```python
from build123d import *
from build123d.topology import SkipClean

# Parameters (mm, degrees)
BOSS_EXTRUDE1_DEPTH                                 = 10.16
CBORE_FOR_0_BINDING_HEAD_MACHINE_SCREW1_D           = 5.08
CBORE_FOR_0_BINDING_HEAD_MACHINE_SCREW1_CBORE_D     = 7.62
CBORE_FOR_0_BINDING_HEAD_MACHINE_SCREW1_CBORE_DEPTH = 1.27
SHELL1_OUTLINE_R                                    = 6.35
SHELL1_DEPTH                                        = 7.62
SHELL1_2_OUTLINE_R                                  = 6.35
SHELL1_2_OUTLINE_R_2                                = 5.08
SHELL1_2_DEPTH                                      = 6.35
CUT_EXTRUDE1_DEPTH                                  = 1.778
CUT_EXTRUDE2_DEPTH                                  = 1.778
CUT_EXTRUDE5_REACH                                  = 157.506
CUT_EXTRUDE6_REACH                                  = 157.506
CUT_EXTRUDE3_DEPTH                                  = 156.506301159
CUT_EXTRUDE3_DEPTH_BACK                             = 156.506301159
SKETCH4_W                                           = 120.65
SKETCH4_H                                           = 5.08
SKETCH5_W                                           = 19.05
SKETCH5_H                                           = 5.08
CUT_EXTRUDE4_DEPTH                                  = 2.54
SKETCH9_W                                           = 47.752
SKETCH9_H                                           = 3.81
CUT_EXTRUDE7_DEPTH                                  = 2.413
FILLET1_R                                           = 1.27
BOSS_EXTRUDE2_DEPTH                                 = 2.54
SKETCH11_W                                          = 40.132
SKETCH11_H                                          = 1.27
CUT_EXTRUDE9_DEPTH                                  = 6.858
SKETCH20_R                                          = 6.35
SKETCH20_R_2                                        = 5.08
CUT_EXTRUDE11_DEPTH                                 = 1.27
BOSS_EXTRUDE4_START                                 = 2.159
BOSS_EXTRUDE4_DEPTH                                 = 2.159
SKETCH36_R                                          = 1.905
CUT_EXTRUDE18_DEPTH                                 = 155.437689597


# Read off the part's stored shape, not the designer's step: Shell1
with BuildPart() as part:
    # Sketch1 → Boss-Extrude1 (new body)
    with BuildSketch(Plane(origin=(0, 0, 0), x_dir=(1, 0, 0), z_dir=(0, 1, 0))):
        with BuildLine():
            Line((0, 0), (133.35, 0))
            Line((133.35, 0), (152.4, 29.21))
            Line((152.4, 29.21), (35.446425772, 29.21))
            ThreePointArc((35.446425772, 29.21), (12.577020299, 22.164640842), (-2.363095051, 3.471333333))
            ThreePointArc((-2.363095051, 3.471333333), (-2.099665053, 1.110662158), (0, 0))
        make_face()
    extrude(amount=BOSS_EXTRUDE1_DEPTH)

    # CBORE for #0 Binding Head Machine Screw1 (through all)
    with Locations(Plane(origin=(0, 10.16, 0), x_dir=(1, 0, 0), z_dir=(0, 1, 0))):
        with Locations((74.100334947, 9.652)):
            CounterBoreHole(CBORE_FOR_0_BINDING_HEAD_MACHINE_SCREW1_D / 2, CBORE_FOR_0_BINDING_HEAD_MACHINE_SCREW1_CBORE_D / 2, CBORE_FOR_0_BINDING_HEAD_MACHINE_SCREW1_CBORE_DEPTH)

    # Shell1 outline → Shell1 (cut)
    with BuildSketch(Plane(origin=(0, 0, 0), x_dir=(1, 0, 0), z_dir=(0, 1, 0))):
        with BuildLine():
            Line((150.743478261, 26.67), (35.446425772, 26.67))
            ThreePointArc((35.446425772, 26.67), (14.006358141, 20.06497579), (0, 2.54))
            Line((0, 2.54), (135.006521739, 2.54))
            Line((135.006521739, 2.54), (150.743478261, 26.67))
        make_face()
        with Locations((74.100334947, 9.652)):
            Circle(SHELL1_OUTLINE_R, mode=Mode.SUBTRACT)
    extrude(amount=SHELL1_DEPTH, mode=Mode.SUBTRACT)

    # Shell1 2 outline → Shell1 2 (cut)
    with BuildSketch(Plane(origin=(0, 0, 0), x_dir=(1, 0, 0), z_dir=(0, 1, 0))):
        with Locations((74.100334947, 9.652)):
            Circle(SHELL1_2_OUTLINE_R)
        with Locations((74.100334947, 9.652)):
            Circle(SHELL1_2_OUTLINE_R_2, mode=Mode.SUBTRACT)
    extrude(amount=SHELL1_2_DEPTH, mode=Mode.SUBTRACT)

    # Sketch2 → Cut-Extrude1 (cut)
    with BuildSketch(Plane.XY):
        Polygon((118.11, 0), (118.11, 5.08), (119.38, 5.08), (119.38, 10.16), (111.76, 10.16), (105.41, 0), align=None)
    extrude(amount=-CUT_EXTRUDE1_DEPTH, mode=Mode.SUBTRACT)

    # Sketch3 → Cut-Extrude2 (cut)
    with BuildSketch(Plane(origin=(0, 0, -29.21), x_dir=(-1, 0, 0), z_dir=(0, 0, -1))):
        Polygon((-138.43, 10.16), (-138.43, 5.08), (-137.16, 5.08), (-137.16, 0), (-124.46, 0), (-130.81, 10.16), align=None)
    extrude(amount=-CUT_EXTRUDE2_DEPTH, mode=Mode.SUBTRACT)

    # Cut-Extrude5: up to this face of the body (flat: up to its plane)
    cut_extrude5_end = Plane(part.part.faces().sort_by_distance((67.503260869, 3.81, -2.54))[0])
    # Sketch7 → Cut-Extrude5 (cut, up to the picked face)
    with BuildSketch(Plane.XY, mode=Mode.PRIVATE) as cut_extrude5_sk1:
        Polygon((135.006521739, 2.979312663), (118.11, 0), (135.006521739, 0), align=None)
    cut_extrude5_tool1 = split(extrude(cut_extrude5_sk1.sketch, amount=-CUT_EXTRUDE5_REACH, mode=Mode.PRIVATE), bisect_by=cut_extrude5_end, keep=Keep.BOTH, mode=Mode.PRIVATE)
    add(cut_extrude5_tool1.solids().sort_by(Axis((129.374348, 0.993104, 0), (0, 0, -1)))[0], mode=Mode.SUBTRACT)

    # Cut-Extrude6: up to this face of the body (flat: up to its plane)
    cut_extrude6_end = Plane(part.part.faces().sort_by_distance((93.094952017, 3.81, -26.67))[0])
    # Sketch8 → Cut-Extrude6 (cut, up to the picked face)
    with BuildSketch(Plane(origin=(0, 0, -29.21), x_dir=(-1, 0, 0), z_dir=(0, 0, -1)), mode=Mode.PRIVATE) as cut_extrude6_sk1:
        Polygon((-152.4, 2.687223186), (-137.16, 0), (-152.4, 0), align=None)
    cut_extrude6_tool1 = split(extrude(cut_extrude6_sk1.sketch, amount=-CUT_EXTRUDE6_REACH, mode=Mode.PRIVATE), bisect_by=cut_extrude6_end, keep=Keep.BOTH, mode=Mode.PRIVATE)
    add(cut_extrude6_tool1.solids().sort_by(Axis((147.32, 0.895741, -29.21), (0, 0, 1)))[0], mode=Mode.SUBTRACT)

    # Sketch4 → Cut-Extrude3 (cut, two sides: drawn at the far end of the back side and taken through both)
    with BuildSketch(Plane.XY.offset(-CUT_EXTRUDE3_DEPTH_BACK)):
        with Locations((57.785, 2.54)):
            Rectangle(SKETCH4_W, SKETCH4_H)
    extrude(amount=CUT_EXTRUDE3_DEPTH + CUT_EXTRUDE3_DEPTH_BACK, mode=Mode.SUBTRACT)

    # Sketch5 → Cut-Extrude4 (cut)
    with BuildSketch(Plane(origin=(0, 0, -29.21), x_dir=(-1, 0, 0), z_dir=(0, 0, -1))):
        with Locations((-127.635, 2.54)):
            Rectangle(SKETCH5_W, SKETCH5_H)
    extrude(amount=-CUT_EXTRUDE4_DEPTH, mode=Mode.SUBTRACT)

    # Sketch9 → Cut-Extrude7 (cut)
    with BuildSketch(Plane(origin=(0, 0, -29.21), x_dir=(-1, 0, 0), z_dir=(0, 0, -1))):
        with Locations((-99.949, 6.985)):
            Rectangle(SKETCH9_W, SKETCH9_H)
    extrude(amount=-CUT_EXTRUDE7_DEPTH, mode=Mode.SUBTRACT)

    # Fillet1
    fillet1_edges = [part.edges().sort_by_distance(p)[0] for p in [
        (145.415, 10.16, -29.21),
        (142.875, 10.16, -14.605),
        (126.365, 10.16, 0),
        (119.38, 10.16, -0.889),
        (55.88, 10.16, 0),
        (-2.099665053, 10.16, -1.110662158),
        (12.577020299, 10.16, -22.164640842),
        (83.128212886, 10.16, -29.21),
        (138.43, 10.16, -28.321),
        (133.35, 6.423611593, 0),
        (152.4, 6.423611593, -29.21),
        (0, 6.35, -2.54),
        (118.745, 5.08, 0),
        (118.11, 2.54, 0),
        (119.38, 7.62, 0),
        (137.16, 2.54, -29.21),
        (137.795, 5.08, -29.21),
        (138.43, 7.62, -29.21),
        (144.78, 1.343611593, -29.21),
        (125.73, 1.343611593, 0),
        (151.57173913, 2.541178448, -27.94),
        (134.17826087, 2.833267924, -1.27),
        (137.16, 5.08, -28.321),
        (118.11, 0, -1.27),
        (118.11, 5.08, -0.889),
        (137.16, 0, -27.94),
    ]]
    fillet(fillet1_edges, radius=FILLET1_R - 0.0001)  # a hair under: the kernel refuses the full size

    # Sketch10 → Boss-Extrude2 (add)
    with BuildSketch(Plane.XZ.offset(-7.62)):
        Polygon((79.883, -21.717), (79.883, -26.67), (112.903, -26.67), (112.903, -19.939), (110.363, -19.939), (110.363, -23.749), (105.283, -23.749), (105.283, -21.717), (102.743, -21.717), (102.743, -23.749), (100.203, -23.749), (100.203, -21.717), (97.663, -21.717), (97.663, -23.749), (95.123, -23.749), (95.123, -21.717), (92.583, -21.717), (92.583, -23.749), (90.043, -23.749), (90.043, -21.717), (87.503, -21.717), (87.503, -23.749), (84.963, -23.749), (84.963, -21.717), align=None)
    extrude(amount=BOSS_EXTRUDE2_DEPTH)

    # Sketch11 → Cut-Extrude9 (cut)
    with BuildSketch(Plane(origin=(0, 0, -26.797), x_dir=(-1, 0, 0), z_dir=(0, 0, -1))):
        with Locations((-99.949, 5.715)):
            Rectangle(SKETCH11_W, SKETCH11_H)
    extrude(amount=-CUT_EXTRUDE9_DEPTH, mode=Mode.SUBTRACT)

    # Sketch20 → Cut-Extrude11 (cut)
    with SkipClean():  # the faces are left unmerged after this step: merging them gives an invalid solid
        with BuildSketch(Plane.XZ.offset(-6.35)):
            with Locations((74.100334947, -9.652)):
                Circle(SKETCH20_R)
            with Locations(Location((74.100334947, -9.652, 0), (0, 0, 90))):
                Circle(SKETCH20_R_2, mode=Mode.SUBTRACT)
        extrude(amount=-CUT_EXTRUDE11_DEPTH, mode=Mode.SUBTRACT)

    # Sketch21 → Boss-Extrude4 (add)
    with BuildSketch(Plane.XZ.offset(-7.62).offset(BOSS_EXTRUDE4_START)):
        with BuildLine():
            Line((74.100334947, -2.54), (74.100334947, -4.572))
            ThreePointArc((74.100334947, -4.572), (73.196935106, -4.652973222), (72.322334947, -4.893311525))
            Line((72.322334947, -4.893311525), (72.322334947, -2.54))
            Line((72.322334947, -2.54), (74.100334947, -2.54))
        make_face()
        with BuildLine():
            Line((74.100334947, -14.732), (74.100334947, -26.67))
            Line((74.100334947, -26.67), (72.322334947, -26.67))
            Line((72.322334947, -26.67), (72.322334947, -14.410688475))
            ThreePointArc((72.322334947, -14.410688475), (73.196935106, -14.651026778), (74.100334947, -14.732))
        make_face()
    extrude(amount=-BOSS_EXTRUDE4_DEPTH)

    # Sketch36 → Cut-Extrude18 (cut, through all)
    with SkipClean():  # the faces are left unmerged after this step: merging them gives an invalid solid
        with BuildSketch(Plane(origin=(0, 10.16, 0), x_dir=(1, 0, 0), z_dir=(0, 1, 0))):
            with Locations(Location((0, 2.54, 0), (0, 0, 270))):
                Circle(SKETCH36_R)
        extrude(amount=-CUT_EXTRUDE18_DEPTH, mode=Mode.SUBTRACT)


solid = part.part
```
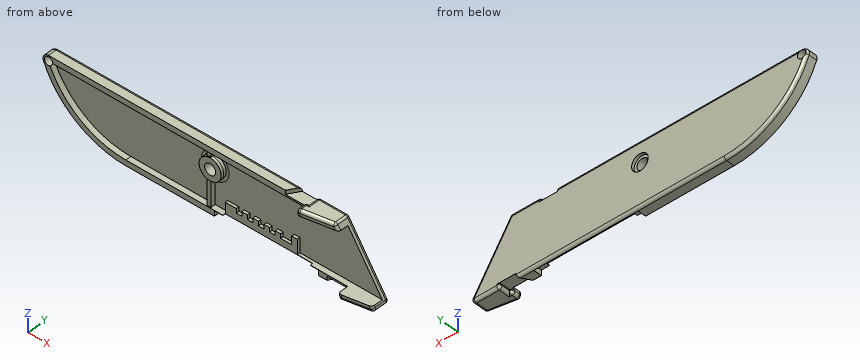
Can you work these out from the model? Positions are in its coordinate system, mm. Round coordinates to 2 decimals unless told otherwise and drop trailing zeros. Loops run counter-clockwise (first coordinate to the right, second up) from the corner with the lowest first, then second, coordinate; pieces in that order, holes last.
Item 1: Please list where these lines run through material, in increasing order: L1, parallel to X at y = 6, z = -7.75; L2, parallel to Z at x = 91, y = 7.5; L3, parallel to Y at x = 33, z = -12.25.
Item 2: Will these pins go through, and if not, where does the flat tip stop? pin 1 Ø1 at (y, z) = (3.5, -2) entering from -X; pin 2 Ø2.5 at (x, z) = (75.5, -10.5) entering from +Y; pin 3 Ø12 at (x, z) = (65.5, -17.5) entering from -Y; pin 4 Ø5 at (x, z) = (0, -2.54) entering from +Y.
Item 3: Suppose I cut it at A-A, the plane x = 52. Write out the boundary of the cut face in (y, z), then the cut area to 3 significant figures.
Reported:
1. L1: x = -0.38 to 2.53, 69.39 to 72.42, 75.78 to 78.81
1. L2: z = -26.8 to -23.75, -2.54 to 0
1. L3: y = 7.62 to 10.16
2. pin 1: stops at x = 118.11
2. pin 2: stops at y = 8.89
2. pin 3: stops at y = 7.62
2. pin 4: stops at y = 10.16
3. outline: (5.08, -29.21) - (8.89, -29.21) arc R1.27 ccw to (10.16, -27.94) - (10.16, -1.27) arc R1.27 ccw to (8.89, 0) - (5.08, 0) - (5.08, -2.54) - (7.62, -2.54) - (7.62, -26.67) - (5.08, -26.67) - close
3. area: 86.4 mm2
